from build123d import *

# Parameters (mm, degrees)
F0_W     = 152.4
F0_H     = 146.05
F1_DEPTH = 5.588
F2_W     = 5.588
F2_H     = 24.13
F2_H_2   = 30.48
F2_H_3   = 24.892
F2_W_2   = 24.892
F2_H_4   = 5.588
F2_W_3   = 30.48
F3_DEPTH = 5.589


with BuildPart() as f1:
    # F0 (on Front) → F1 (new body)
    with BuildSketch(Plane.XZ):
        with Locations((0, -1.799165)):
            Rectangle(F0_W, F0_H)
    extrude(amount=F1_DEPTH)

    # F2 (on face) → F3 (cut, through all)
    with BuildSketch(Plane.XZ.offset(5.588)):
        with Locations((-73.406, 59.160835)):
            Rectangle(F2_W, F2_H)
        with Locations((-73.406, 1.375835)):
            Rectangle(F2_W, F2_H_2)
        with Locations((-73.406, -56.790165)):
            Rectangle(F2_W, F2_H_3)
        with Locations((-58.166, -72.030165)):
            Rectangle(F2_W_2, F2_H_4)
        with Locations((-73.406, -72.030165)):
            Rectangle(F2_W, F2_H_4)
        with Locations((0, -72.030165)):
            Rectangle(F2_W_3, F2_H_4)
        with Locations((58.166, -72.030165)):
            Rectangle(F2_W_2, F2_H_4)
        with Locations((73.406, -72.030165)):
            Rectangle(F2_W, F2_H_4)
        with Locations((73.406, -56.790165)):
            Rectangle(F2_W, F2_H_3)
        with Locations((73.406, 1.375835)):
            Rectangle(F2_W, F2_H_2)
        with Locations((73.406, 59.160835)):
            Rectangle(F2_W, F2_H)
    extrude(amount=-F3_DEPTH, mode=Mode.SUBTRACT)


solid = f1.part
Input: part model. Units: mm. Frame: model coordinates. A direction names the side the tool comes from. Give positions to 0.01 mm unless a question says otherwise; leave off trailing zeros. Write each loop counter-clockwise with the first axis right and the second up, starting at its lowest first coordinate (ties: lowest second). Pieces come first, ordered by that corner, then holes.
Q1. Section B-B, the plane z = -63. Output: boundary loops of the cut face in (x, y), plus the area to 3 significant figures.
Q2. Pull-direction query (X, two-part tool) for faces 6 (the face through (30, -3, -74.824)), 7 (the face through (45.72, -3, -72)), 8 (the face through (-70.612, -3, 1)), 9 (the face through (15.24, -3, -72)); classes: pulls with the +X half, pulls with the -X half, needs draft (parallel to the pull), parting line crosses it, or undercut.
Q3. Material intervals for probe 1 along X at (y, z) = (-1.6, -63.5); probe 2 along Z at (x, y) = (-64, -1.3), sorted ascending.
Q4. Section C-C, the plane x = 63. Output: boundary loops of the cut face in (y, z), plus the area to 3 significant figures.
Q5. Set-up query: faces 1 (the face through (70.612, -3, -57)), 2 (the face through (-70.612, -3, 59)), 3 (the face through (-70.612, -3, -57)), 4 (the face through (73, -3, -13.864)), 5 (the face through (73, -3, 47.096)). Return all of +Z, -Z, +X, -X, +Y, -Y with unobstructed straight access to the full face (end or side cutting, diameter ignored); none if empty.
Q6. Section A-A, the plane y = -1.2. Output: boundary loops of the cut face in (x, z), plus the area to 3 significant figures.
Q7. First-contact query: P1, Ø1.7, axis at y = -4, z = 2.5, coming from the -X side; P2, Ø1.7, axis at x = 74, y = -2, coming from the +Z side; P3, Ø3, axis at x = -74, y = -2.5, coming from the -Z side; P4, Ø1, axis at x = 14, z = 29, coming from the +Y side. Flat tips, straight axial feed; report the tip coordinate or a pass-through.
Filled in:
1. outline: (-70.61, -5.59) - (70.61, -5.59) - (70.61, 0) - (-70.61, 0) - close
1. area: 789 mm2
2. face 6: needs draft
2. face 7: pulls with the +X half
2. face 8: pulls with the -X half
2. face 9: undercut
3. probe 1: x = -70.61 to 70.61
3. probe 2: z = -69.24 to 71.23
4. outline: (-5.59, -69.24) - (0, -69.24) - (0, 71.23) - (-5.59, 71.23) - close
4. area: 785 mm2
5. face 1: -Z, +X, +Y, -Y
5. face 2: +Z, -X, +Y, -Y
5. face 3: -Z, -X, +Y, -Y
5. face 4: +X, +Y, -Y
5. face 5: +Z, +X, +Y, -Y
6. outline: (-76.2, -44.34) - (-70.61, -44.34) - (-70.61, -69.24) - (-45.72, -69.24) - (-45.72, -74.82) - (-15.24, -74.82) - (-15.24, -69.24) - (15.24, -69.24) - (15.24, -74.82) - (45.72, -74.82) - (45.72, -69.24) - (70.61, -69.24) - (70.61, -44.34) - (76.2, -44.34) - (76.2, -13.86) - (70.61, -13.86) - (70.61, 16.62) - (76.2, 16.62) - (76.2, 47.1) - (70.61, 47.1) - (70.61, 71.23) - (-70.61, 71.23) - (-70.61, 47.1) - (-76.2, 47.1) - (-76.2, 16.62) - (-70.61, 16.62) - (-70.61, -13.86) - (-76.2, -13.86) - close
6. area: 20,900 mm2
7. P1: stops at x = -70.61
7. P2: stops at z = 47.1
7. P3: stops at z = -44.34
7. P4: stops at y = 0
